from build123d import *

# Parameters (mm, degrees)
SKETCH1_R           = 3
BOSS_EXTRUDE1_DEPTH = 2.8
FILLET1_R           = 4


with BuildPart() as part:
    # Sketch1 → Boss-Extrude1 (new body)
    with BuildSketch(Plane(origin=(0, 0, 0), x_dir=(1, 0, 0), z_dir=(0, 1, 0))):
        with BuildLine():
            Line((-354.423555473, -2063.72823662), (-365.363735679, -2118.72823662))
            ThreePointArc((-365.363735679, -2118.72823662), (0, -2150), (365.363735679, -2118.72823662))
            Line((365.363735679, -2118.72823662), (354.423555473, -2063.72823662))
            Line((354.423555473, -2063.72823662), (-354.423555473, -2063.72823662))
        make_face()
        with Locations((0, -2088.423050098)):
            Circle(SKETCH1_R, mode=Mode.SUBTRACT)
        with Locations((110, -2088.423050098)):
            Circle(SKETCH1_R, mode=Mode.SUBTRACT)
        with Locations((220, -2088.423050098)):
            Circle(SKETCH1_R, mode=Mode.SUBTRACT)
        with Locations((330, -2088.423050098)):
            Circle(SKETCH1_R, mode=Mode.SUBTRACT)
        with Locations((-110, -2088.423050098)):
            Circle(SKETCH1_R, mode=Mode.SUBTRACT)
        with Locations((-220, -2088.423050098)):
            Circle(SKETCH1_R, mode=Mode.SUBTRACT)
        with Locations((-330, -2088.423050098)):
            Circle(SKETCH1_R, mode=Mode.SUBTRACT)
    extrude(amount=BOSS_EXTRUDE1_DEPTH)

    # Fillet1
    fillet1_edges = [part.edges().sort_by_distance(p)[0] for p in [
        (365.363735679, 1.4, 2118.72823662),
        (-365.363735679, 1.4, 2118.72823662),
        (-354.423555473, 1.4, 2063.72823662),
        (354.423555473, 1.4, 2063.72823662),
    ]]
    fillet(fillet1_edges, radius=FILLET1_R)


solid = part.part
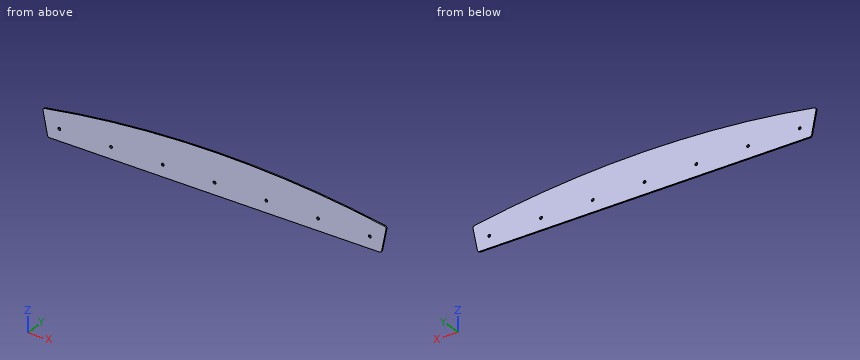
The model under review builds one solid part; all positions refer to its coordinate system, in mm. Give positions to 0.01 mm unless a question says otherwise; leave off trailing zeros. Loops run counter-clockwise (first coordinate to the right, second up) from the corner with the lowest first, then second, coordinate; pieces in that order, holes last. Notation, with made-up numbers: (5.5, -30) -> (46.5, -30) arc R35 cw to (46.5, 6) -> close; hole circle Ø11 at (-8.75, -35.75). An arc over 180 degrees is marked (long way). Write each question's results on one line, items separated by ' | '.
1) Take a section at C-C, the plane x = -236. Give the boundary of the cut face in (y, z), plus the area to 3 significant figures.
Conclusion:
outline: (0, 2063.73) -> (2.8, 2063.73) -> (2.8, 2137.01) -> (0, 2137.01) -> close | area: 205 mm^2
2) Insertion check: pin 1 Ø2 at (x, z) = (-270, 2128) entering from -Y. The pin has a flat end and moves straight along its axis. Give the tip position at first contact, or say it passes through.
Conclusion:
pin 1: stops at y = 0
3) Take a section at B-B, the plane z = 2073. Give the boundary of the cut face in (x, y), plus the area to 3 significant figures.
Conclusion:
outline: (-356.27, 0) -> (356.27, 0) -> (356.27, 2.8) -> (-356.27, 2.8) -> close | area: 2,000 mm^2
4) Take a section at A-A, the plane y = 1.4. Give the boundary of the cut face in (x, z), plus the area to 3 significant figures.
Conclusion:
outline: (-364.56, 2114.7) -> (-355.06, 2066.95) arc R4 ccw to (-351.14, 2063.73) -> (351.14, 2063.73) arc R4 ccw to (355.06, 2066.95) -> (364.56, 2114.7) arc R4 ccw to (361.31, 2119.42) arc R2150 ccw to (-361.31, 2119.42) arc R4 ccw to start; hole circle Ø6 at (-330, 2088.42); hole circle Ø6 at (-220, 2088.42); hole circle Ø6 at (-110, 2088.42); hole circle Ø6 at (0, 2088.42); hole circle Ø6 at (110, 2088.42); hole circle Ø6 at (220, 2088.42); hole circle Ø6 at (330, 2088.42) | area: 54,600 mm^2
5) For line 1 along Z through (x, y) = (110, 2.05); line 2 along Z through (x, y) = (-222.5, 1.75); line 3 along Z through (x, y) = (70.5, 0.6), list the stretches that pass through material, from the lowest coordinate up. Write a range as from..to.
Conclusion:
line 1: z = 2063.73..2085.42, 2091.42..2147.18 | line 2: z = 2063.73..2086.76, 2090.08..2138.46 | line 3: z = 2063.73..2148.84
